Check sheet for the modelled part. Datum: model origin and axes. Units: mm. Round coordinates to 2 decimals unless told otherwise and drop trailing zeros. Loops run counter-clockwise (first coordinate to the right, second up) from the corner with the lowest first, then second, coordinate; pieces in that order, holes last. Notation, with made-up numbers: (76, 29) -> (127, 29) arc R21 cw to (127, 65) -> close; hole circle Ø7 at (6.25, 1). An arc over 180 degrees is marked (long way). Return JSON: item names as keys, results as strings.
from build123d import *

# Parameters (mm, degrees)
CROQUIS1_R              = 4.5
SALIENTE_EXTRUIR1_DEPTH = 9
CHAFL_N1_SIZE           = 0.3
CHAFL_N2_SIZE           = 0.3
CROQUIS2_R              = 1.55
CORTAR_EXTRUIR1_DEPTH   = 9


with BuildPart() as part:
    # Croquis1 → Saliente-Extruir1 (new body)
    with BuildSketch(Plane(origin=(0, 0, 0), x_dir=(1, 0, 0), z_dir=(0, 1, 0))):
        with Locations(Location((0, 0, 0), (0, 0, 270))):
            Circle(CROQUIS1_R)
    extrude(amount=SALIENTE_EXTRUIR1_DEPTH)

    # Chaflán1
    chafl_n1_edges = [part.edges().sort_by_distance(p)[0] for p in [
        (0, 9, -4.5),
    ]]
    chamfer(chafl_n1_edges, length=CHAFL_N1_SIZE)

    # Chaflán2
    chafl_n2_edges = [part.edges().sort_by_distance(p)[0] for p in [
        (0, 0, -4.5),
    ]]
    chamfer(chafl_n2_edges, length=CHAFL_N2_SIZE)

    # Croquis2 → Cortar-Extruir1 (cut)
    with BuildSketch(Plane(origin=(0, 9, 0), x_dir=(1, 0, 0), z_dir=(0, 1, 0))):
        with Locations(Location((0, 0, 0), (0, 0, 270))):
            Circle(CROQUIS2_R)
    extrude(amount=-CORTAR_EXTRUIR1_DEPTH, mode=Mode.SUBTRACT)


solid = part.part
Q1. Material ranges on line 1 (X direction, y = 1.5, z = 0); line 2 (Z direction, x = 0.75, y = 5.25); line 3 (Z direction, x = -1, y = 7), recorded low to high.
Results list:
{"line 1": "-4.5 to -1.55, 1.55 to 4.5", "line 2": "-4.44 to -1.36, 1.36 to 4.44", "line 3": "-4.39 to -1.18, 1.18 to 4.39"}
Q2. Go/stop test with flat-tipped pins: pin 1 (1.5 mm diameter, centred on y = 6.5, z = 2.5, fed in from +X); pin 2 (3 mm diameter, centred on y = 2.5, z = 2.5, fed in from +X); pin 3 (3 mm diameter, centred on x = -1, y = 4, fed in from -Z); pin 4 (1 mm diameter, centred on x = -2, y = 5, fed in from +Z). Record where each tip stops, or that it passes through.
Results list:
{"pin 1": "x = 4.15", "pin 2": "x = 4.39", "pin 3": "z = -4.5", "pin 4": "z = 4.24"}
Q3. Section check A-A (z = 0). Record the boundary of the cut face in (x, y).
Results list:
{"outline": "(-4.5, 0.3) -> (-4.2, 0) -> (-1.55, 0) -> (-1.55, 9) -> (-4.2, 9) -> (-4.5, 8.7) -> close; (1.55, 0) -> (4.2, 0) -> (4.5, 0.3) -> (4.5, 8.7) -> (4.2, 9) -> (1.55, 9) -> close"}
Q4. Draft check along Z on faces 1 (the cylindrical face through (1.352, 4.441, 4.292)), 2 (the flat face through (0, 0, 2)), 3 (the cylindrical face through (0.466, 4.563, 1.478)). Enter one of: released by +Z, released by -Z, zero draft, split by the parting line, or undercut.
Results list:
{"face 1": "split by the parting line", "face 2": "zero draft", "face 3": "undercut"}
Q5. Section check B-B (y = 7.75). Record the boundary of the cut face in (x, z).
Results list:
{"outline": "circle Ø9 at (0, 0); hole circle Ø3.1 at (0, 0)"}
